```python
from build123d import *

# Parameters (mm, degrees)
SKIZZE4_W                       = 47.8
SKIZZE4_H                       = 37.511655438
AUFSATZ_LINEAR_AUSTRAGEN2_DEPTH = 2
SKIZZE5_W                       = 47.8
SKIZZE5_H                       = 3.6
SKIZZE5_H_2                     = 3.4
AUFSATZ_LINEAR_AUSTRAGEN3_DEPTH = 12
SKIZZE6_R                       = 1
SCHNITT_LINEAR_AUSTRAGEN1_DEPTH = 19
SKIZZE8_W                       = 47.8
SKIZZE8_H                       = 12
AUFSATZ_LINEAR_AUSTRAGEN4_DEPTH = 3
SKIZZE9_W                       = 47.8
SKIZZE9_H                       = 12
AUFSATZ_LINEAR_AUSTRAGEN5_DEPTH = 3
SKIZZE10_W                      = 12
SKIZZE10_H                      = 43.511655438
AUFSATZ_LINEAR_AUSTRAGEN6_DEPTH = 0.5
SKIZZE11_W                      = 12
SKIZZE11_H                      = 43.511655438
AUFSATZ_LINEAR_AUSTRAGEN7_DEPTH = 0.5
SKIZZE12_R                      = 1.5
SCHNITT_LINEAR_AUSTRAGEN2_DEPTH = 9
SCHNITT_LINEAR_START            = -9
SKIZZE13_R                      = 1.5
SCHNITT_LINEAR_AUSTRAGEN3_DEPTH = 9
SKIZZE14_R                      = 2.35
SCHNITT_LINEAR_AUSTRAGEN4_DEPTH = 4
SCHNITT_LINEAR_START_2          = -4
SKIZZE15_R                      = 2.35
SCHNITT_LINEAR_AUSTRAGEN5_DEPTH = 4
VERRUNDUNG3_R                   = 1
VERRUNDUNG4_R                   = 1
VERRUNDUNG5_R                   = 7
SKIZZE17_R                      = 2.35
SCHNITT_LINEAR_AUSTRAGEN6_DEPTH = 4
SKIZZE18_R                      = 1.5
SCHNITT_LINEAR_AUSTRAGEN7_DEPTH = 14
SKIZZE19_R                      = 1.5
SCHNITT_LINEAR_AUSTRAGEN8_DEPTH = 14


with BuildPart() as part:
    # Skizze4 → Aufsatz-Linear austragen2 (new body)
    with BuildSketch(Plane.XY):
        with Locations((11.372253432, 7.302337754)):
            Rectangle(SKIZZE4_W, SKIZZE4_H)
    extrude(amount=AUFSATZ_LINEAR_AUSTRAGEN2_DEPTH)

    # Skizze5 → Aufsatz-Linear austragen3 (add)
    with BuildSketch(Plane(origin=(0, 0, 0), x_dir=(-1, 0, 0), z_dir=(0, 0, -1))):
        with Locations((-11.372253432, 24.258165473)):
            Rectangle(SKIZZE5_W, SKIZZE5_H)
        with Locations((-11.372253432, -9.753489965)):
            Rectangle(SKIZZE5_W, SKIZZE5_H_2)
    extrude(amount=-AUFSATZ_LINEAR_AUSTRAGEN3_DEPTH)

    # Skizze6 → Schnitt-Linear austragen1 (cut)
    with BuildSketch(Plane(origin=(0, 0, 0), x_dir=(-1, 0, 0), z_dir=(0, 0, -1))):
        with Locations((2.527746568, 23.483879087)):
            Circle(SKIZZE6_R)
        with Locations((2.540359159, -9.04853229)):
            Circle(SKIZZE6_R)
    extrude(amount=-SCHNITT_LINEAR_AUSTRAGEN1_DEPTH, mode=Mode.SUBTRACT)

    # Skizze8 → Aufsatz-Linear austragen4 (add)
    with BuildSketch(Plane(origin=(0, 26.058165473, 0), x_dir=(1, 0, 0), z_dir=(0, 1, 0))):
        with Locations((11.372253432, -6)):
            Rectangle(SKIZZE8_W, SKIZZE8_H)
    extrude(amount=AUFSATZ_LINEAR_AUSTRAGEN4_DEPTH)

    # Skizze9 → Aufsatz-Linear austragen5 (add)
    with BuildSketch(Plane.XZ.offset(11.453489965)):
        with Locations((11.372253432, 6)):
            Rectangle(SKIZZE9_W, SKIZZE9_H)
    extrude(amount=AUFSATZ_LINEAR_AUSTRAGEN5_DEPTH)

    # Skizze10 → Aufsatz-Linear austragen6 (add)
    with BuildSketch(Plane.ZY.offset(12.527746568)):
        with Locations((6, 7.302337754)):
            Rectangle(SKIZZE10_W, SKIZZE10_H)
    extrude(amount=AUFSATZ_LINEAR_AUSTRAGEN6_DEPTH)

    # Skizze11 → Aufsatz-Linear austragen7 (add)
    with BuildSketch(Plane(origin=(35.272253432, 0, 0), x_dir=(0, 0, -1), z_dir=(1, 0, 0))):
        with Locations((-6, 7.302337754)):
            Rectangle(SKIZZE11_W, SKIZZE11_H)
    extrude(amount=AUFSATZ_LINEAR_AUSTRAGEN7_DEPTH)

    # Skizze12 → Schnitt-Linear austragen2 (cut)
    with BuildSketch(Plane.ZY.offset(13.027746568)):
        with Locations(Location((6, 25.858165473, 0), (0, 0, 270))):
            Circle(SKIZZE12_R)
    extrude(amount=-SCHNITT_LINEAR_AUSTRAGEN2_DEPTH, mode=Mode.SUBTRACT)

    # Skizze13 → Schnitt-Linear austragen3 (cut)
    with BuildSketch(Plane(origin=(35.772253432, 0, 0), x_dir=(0, 0, -1), z_dir=(1, 0, 0)).offset(SCHNITT_LINEAR_START)):
        with Locations(Location((-6, 25.858165473, 0), (0, 0, 270))):
            Circle(SKIZZE13_R)
    extrude(amount=SCHNITT_LINEAR_AUSTRAGEN3_DEPTH, mode=Mode.SUBTRACT)

    # Skizze14 → Schnitt-Linear austragen4 (cut)
    with BuildSketch(Plane.ZY.offset(13.027746568)):
        with Locations(Location((6, 25.858165473, 0), (0, 0, 270))):
            Circle(SKIZZE14_R)
    extrude(amount=-SCHNITT_LINEAR_AUSTRAGEN4_DEPTH, mode=Mode.SUBTRACT)

    # Skizze15 → Schnitt-Linear austragen5 (cut)
    with BuildSketch(Plane(origin=(35.772253432, 0, 0), x_dir=(0, 0, -1), z_dir=(1, 0, 0)).offset(SCHNITT_LINEAR_START_2)):
        with Locations(Location((-6, 25.858165473, 0), (0, 0, 270))):
            Circle(SKIZZE15_R)
    extrude(amount=SCHNITT_LINEAR_AUSTRAGEN5_DEPTH, mode=Mode.SUBTRACT)

    # Verrundung3
    # the kernel refuses this fillet: 1 mm, written as the material it takes off along each edge
    with BuildSketch(Plane(origin=(35.772253432, 29.058165473, 14.5), x_dir=(-1, 0, 0), z_dir=(0, 0, -1))) as verrundung3_piece_1:
        with BuildLine():
            CenterArc((VERRUNDUNG3_R, -VERRUNDUNG3_R), VERRUNDUNG3_R, 90, 90)
            Line((0, -VERRUNDUNG3_R), (0, 0))
            Line((0, 0), (VERRUNDUNG3_R, 0))
        make_face()
    extrude(amount=17, mode=Mode.SUBTRACT)

    # Verrundung4
    # the kernel refuses this fillet: 1 mm, written as the material it takes off along each edge
    with BuildSketch(Plane(origin=(-13.027746568, 29.058165473, 14.5), x_dir=(1, 0, 0), z_dir=(0, 0, -1))) as verrundung4_piece_1:
        with BuildLine():
            CenterArc((VERRUNDUNG4_R, VERRUNDUNG4_R), VERRUNDUNG4_R, 180, 90)
            Line((0, VERRUNDUNG4_R), (0, 0))
            Line((0, 0), (VERRUNDUNG4_R, 0))
        make_face()
    extrude(amount=17, mode=Mode.SUBTRACT)

    # Verrundung5
    verrundung5_edges = [part.edges().sort_by_distance(p)[0] for p in [
        (35.772253432, -14.453489965, 6),
        (-13.027746568, -14.453489965, 6),
    ]]
    fillet(verrundung5_edges, radius=VERRUNDUNG5_R)

    # Skizze17 → Schnitt-Linear austragen6 (cut)
    with BuildSketch(Plane.XY.offset(12)):
        with Locations((11.372253432, -11.253489965)):
            Circle(SKIZZE17_R)
        with Locations((11.372253432, 25.858165473)):
            Circle(SKIZZE17_R)
    extrude(amount=-SCHNITT_LINEAR_AUSTRAGEN6_DEPTH, mode=Mode.SUBTRACT)

    # Skizze18 → Schnitt-Linear austragen7 (cut)
    with BuildSketch(Plane.XY.offset(8)):
        with Locations((11.372253432, -11.253489965)):
            Circle(SKIZZE18_R)
        with Locations((11.372253432, 25.858165473)):
            Circle(SKIZZE18_R)
    extrude(amount=-SCHNITT_LINEAR_AUSTRAGEN7_DEPTH, mode=Mode.SUBTRACT)

    # Skizze19 → Schnitt-Linear austragen8 (cut)
    with BuildSketch(Plane.XY.offset(2)):
        with Locations((-11.027746568, -3.053489965)):
            Circle(SKIZZE19_R)
        with Locations((33.772253432, 17.458165473)):
            Circle(SKIZZE19_R)
    extrude(amount=-SCHNITT_LINEAR_AUSTRAGEN8_DEPTH, mode=Mode.SUBTRACT)


solid = part.part
```
For this review, take the finished solid that the model builds, in its own axes (mm). A direction names the side the tool comes from. Round coordinates to 2 decimals unless told otherwise and drop trailing zeros. Loops run counter-clockwise (first coordinate to the right, second up) from the corner with the lowest first, then second, coordinate; pieces in that order, holes last.
(1) Wall thickness on line 1 along X through (y, z) = (13, 9); line 2 along Y through (x, z) = (13.5, 3); line 3 along Y through (x, z) = (12.5, 1.75): over which ranges is each line inside the solid? List them lowest first.
Returned:
line 1: x = -13.03 to -12.53, 35.27 to 35.77
line 2: y = -14.45 to -8.05, 22.46 to 29.06
line 3: y = -14.45 to -12.24, -10.26 to 24.87, 26.85 to 29.06
(2) We need section A-A (x = 27.5). Give the boundary of the cut face in (y, z), plus the area to 3 significant figures.
Returned:
outline: (-14.45, 0) - (29.06, 0) - (29.06, 12) - (22.46, 12) - (22.46, 2) - (-8.05, 2) - (-8.05, 12) - (-14.45, 12) - close; hole circle Ø3 at (25.86, 6)
area: 210 mm2
(3) Clearance check with flat-ended pins moving along their axes: P1, Ø15.5, axis at x = 5.5, y = 4, coming from the +Z side; P2, Ø0.9, axis at y = 26.5, z = 6, coming from the -X side; P3, Ø1.8, axis at x = 33.77, y = 17.46, coming from the +Z side; P4, Ø4, axis at y = 25.86, z = 6, coming from the -X side. State where each tip first meets the part, or that it passes through.
Returned:
P1: stops at z = 2
P2: stops at x = -4.03
P3: passes through
P4: stops at x = -9.03
(4) Mouldability with a two-part tool opening along Z and no side actions: class faces 1 (the flat face through (13, 23, 12)), 2 (the flat face through (11, 29.058, 6)), 3 (the flat face through (31.772, 24, 6)) as released by +Z, released by -Z, zero draft, split by the parting line, or undercut.
Returned:
face 1: released by +Z
face 2: zero draft
face 3: undercut
(5) We need section D-D (z = 6). State how many separate pieces and enclosed holes the cut face has, plus the area to 3 significant figures.
Returned:
separate pieces: 1
enclosed holes: 4
area: 555 mm2
(6) We need section B-B (z = 10.25). Give the boundary of the cut face in (x, y), plus the area to 3 significant figures.
Returned:
outline: (-13.03, -7.45) arc R7 ccw to (-6.03, -14.45) - (28.77, -14.45) arc R7 ccw to (35.77, -7.45) - (35.77, 28.06) arc R1 ccw to (34.77, 29.06) - (-12.03, 29.06) arc R1 ccw to (-13.03, 28.06) - close; hole (-12.53, -8.05) - (-2.64, -8.05) arc R1 ccw (long way) to (-2.44, -8.05) - (35.27, -8.05) - (35.27, 22.46) - (-12.53, 22.46) - close; hole circle Ø2 at (-2.53, 23.48); hole circle Ø4.7 at (11.37, -11.25); hole circle Ø4.7 at (11.37, 25.86)
area: 602 mm2
(7) Tool access review of faces 4 (the flat face through (11, -13, 8)), 5 (the flat face through (26.772, 26, 6)), 6 (the cylindrical face through (-6.563, 24.427, 6.451)): name each direction out of +Z, -Z, +X, -X, +Y, -Y from which nothing blocks a thin tool from reaching the whole face with its end or side.
Returned:
face 4: +Z
face 5: +X
face 6: -X
(8) We need section C-C (x = 20). Give the boundary of the cut face in (y, z), plus the area to 3 significant figures.
Returned:
outline: (-14.45, 0) - (29.06, 0) - (29.06, 12) - (22.46, 12) - (22.46, 2) - (-8.05, 2) - (-8.05, 12) - (-14.45, 12) - close
area: 217 mm2
